Could you check a few things on this model? Use its own coordinates, in mm. Coordinates: 2 decimals unless noted, no trailing zeros. Order: outer loops, then holes, each group sorted by start corner. A loop starts at its lowest first (then second) coordinate and runs counter-clockwise, first axis right, second up. Notation, with made-up numbers: (86, 8) - (112, 8) arc R38 ccw to (112, 47) - close; hole circle Ø7 at (79.5, -3.75). An arc over 180 degrees is marked (long way). One line per item, written item: value.
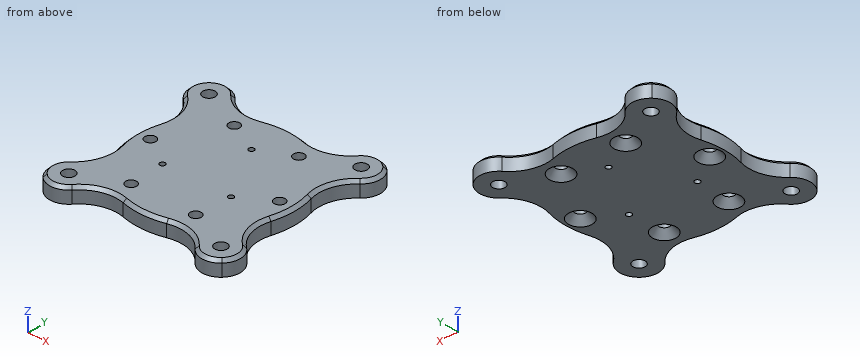
from build123d import *

# Parameters (mm, degrees)
SKETCH1_R                                      = 53.975
BOSS_EXTRUDE1_DEPTH                            = 6.35
CSK_FOR_8_FLAT_HEAD_MACHINE_SCREW1_D           = 4.4958
CSK_FOR_8_FLAT_HEAD_MACHINE_SCREW1_CSINK_D     = 9.7575878
CSK_FOR_8_FLAT_HEAD_MACHINE_SCREW1_CSINK_ANGLE = 82
CIRPATTERN1_COUNT                              = 6
F_10_CLEARANCE_HOLE1_D                         = 5.1054
CIRPATTERN2_COUNT                              = 4
F_4_40_TAPPED_HOLE1_D                          = 2.2606
CIRPATTERN3_COUNT                              = 3
CUT_EXTRUDE2_DEPTH                             = 77.59584682
CIRPATTERN4_COUNT                              = 4
CHAMFER1_SIZE                                  = 1.27


with BuildPart() as part:
    # Sketch1 → Boss-Extrude1 (new body)
    with BuildSketch(Plane.XY):
        Circle(SKETCH1_R)
    extrude(amount=BOSS_EXTRUDE1_DEPTH)

    # CSK for #8 Flat Head Machine Screw1 (through all)
    with Locations(Plane(origin=(0, 0, 0), x_dir=(-1, 0, 0), z_dir=(0, 0, -1))):
        with Locations((-13.49375, 23.371860585)):
            csk_for_8_flat_head_machine_screw1 = CounterSinkHole(CSK_FOR_8_FLAT_HEAD_MACHINE_SCREW1_D / 2, CSK_FOR_8_FLAT_HEAD_MACHINE_SCREW1_CSINK_D / 2, counter_sink_angle=CSK_FOR_8_FLAT_HEAD_MACHINE_SCREW1_CSINK_ANGLE)

    # CirPattern1: CSK for #8 Flat Head Machine Screw1 ×6 about axis
    cirpattern1_axis = Axis((0, 0, 0), (0, 0, 1))
    for i in range(1, CIRPATTERN1_COUNT):
        add(csk_for_8_flat_head_machine_screw1.rotate(cirpattern1_axis, i * 360 / CIRPATTERN1_COUNT), mode=Mode.SUBTRACT)

    # #10 Clearance Hole1 (through all)
    with Locations(Plane.XY.offset(6.35)):
        with Locations((31.75, 31.75)):
            f_10_clearance_hole1 = Hole(F_10_CLEARANCE_HOLE1_D / 2)

    # CirPattern2: #10 Clearance Hole1 ×4 about axis
    cirpattern2_axis = Axis((0, 0, 0), (0, 0, 1))
    for i in range(1, CIRPATTERN2_COUNT):
        add(f_10_clearance_hole1.rotate(cirpattern2_axis, i * 360 / CIRPATTERN2_COUNT), mode=Mode.SUBTRACT)

    # #4-40 Tapped Hole1 (through all)
    with Locations(Plane.XY.offset(6.35)):
        with Locations((0, 16.51)):
            f_4_40_tapped_hole1 = Hole(F_4_40_TAPPED_HOLE1_D / 2)

    # CirPattern3: #4-40 Tapped Hole1 ×3 about axis
    cirpattern3_axis = Axis((0, 0, 0), (0, 0, 1))
    for i in range(1, CIRPATTERN3_COUNT):
        add(f_4_40_tapped_hole1.rotate(cirpattern3_axis, i * 360 / CIRPATTERN3_COUNT), mode=Mode.SUBTRACT)

    # Sketch9 → Cut-Extrude2 (cut, through all)
    with BuildSketch(Plane(origin=(0, 0, 0), x_dir=(-1, 0, 0), z_dir=(0, 0, -1))):
        with BuildLine():
            Line((-37.362660076, 37.362660076), (-38.166088515, 38.166088515))
            ThreePointArc((-38.166088515, 38.166088515), (0, 53.975), (38.166088515, 38.166088515))
            Line((38.166088515, 38.166088515), (37.362660076, 37.362660076))
            ThreePointArc((37.362660076, 37.362660076), (31.392484898, 39.679444445), (25.65502333, 36.834797503))
            ThreePointArc((25.65502333, 36.834797503), (18.130045784, 31.830282128), (9.09329402, 31.74322611))
            ThreePointArc((9.09329402, 31.74322611), (0, 33.02), (-9.09329402, 31.74322611))
            ThreePointArc((-9.09329402, 31.74322611), (-18.130045784, 31.830282128), (-25.65502333, 36.834797503))
            ThreePointArc((-25.65502333, 36.834797503), (-31.392484898, 39.679444445), (-37.362660076, 37.362660076))
        make_face()
    cut_extrude2 = extrude(amount=-CUT_EXTRUDE2_DEPTH, mode=Mode.SUBTRACT)

    # CirPattern4: Cut-Extrude2 ×4 about axis
    cirpattern4_axis = Axis((0, 0, 0), (0, 0, 1))
    for i in range(1, CIRPATTERN4_COUNT):
        add(cut_extrude2.rotate(cirpattern4_axis, i * 360 / CIRPATTERN4_COUNT), mode=Mode.SUBTRACT)

    # Chamfer1
    chamfer1_edges = [part.edges().sort_by_distance(p)[0] for p in [
        (37.362660076, 37.362660076, 6.35),
        (-37.362660076, 37.362660076, 6.35),
        (-18.130045784, 31.830282128, 6.35),
        (0, 33.02, 6.35),
        (18.130045784, 31.830282128, 6.35),
        (37.362660076, -37.362660076, 6.35),
        (31.830282128, 18.130045784, 6.35),
        (33.02, 0, 6.35),
        (31.830282128, -18.130045784, 6.35),
        (-37.362660076, -37.362660076, 6.35),
        (18.130045784, -31.830282128, 6.35),
        (0, -33.02, 6.35),
        (-18.130045784, -31.830282128, 6.35),
        (-31.830282128, -18.130045784, 6.35),
        (-33.02, 0, 6.35),
        (-31.830282128, 18.130045784, 6.35),
    ]]
    chamfer(chamfer1_edges, length=CHAMFER1_SIZE)


solid = part.part
Item 1: I'm going to push flat-ended pins straight in: pin 1 Ø4.5 at (x, y) = (-31.75, 31.75) entering from +Z; pin 2 Ø1.5 at (x, z) = (-9, 5) entering from +Y; pin 3 Ø1.5 at (x, z) = (7.5, 0.5) entering from +Y; pin 4 Ø6 at (x, y) = (-26.99, 0) entering from -Z. Where does each tip first touch, or does it pass through?
Conclusion:
pin 1: through
pin 2: y = 31.97
pin 3: y = 32.32
pin 4: z = 2.16
Item 2: I want a section at B-B on z = 1.75. Give the number of separate pieces and of enclosed holes in the cut face, then the cut area to 3 significant figures.
Conclusion:
separate pieces: 1
enclosed holes: 13
area: 4,420 mm²
Item 3: I want a section at A-A on x = 0. Please give me the cut outline in (y, z).
Conclusion:
outline: (-33.02, 0) - (15.38, 0) - (15.38, 6.35) - (-31.75, 6.35) - (-33.02, 5.08) - close; (17.64, 0) - (33.02, 0) - (33.02, 5.08) - (31.75, 6.35) - (17.64, 6.35) - close
Item 4: If I drill on probe 1 along Y at (x, z) = (-30, 1); probe 2 along Y at (x, z) = (-30, 1.75); probe 3 along X at (y, z) = (30.5, 3.75), over which ranges is the centre line in solid material (lowest first)?
Conclusion:
probe 1: -39.49 to -33.61, -29.89 to -2.65, 2.65 to 29.89, 33.61 to 39.49
probe 2: -39.49 to -33.61, -29.89 to -1.48, 1.48 to 29.89, 33.61 to 39.49
probe 3: -39.59 to -33.98, -29.52 to 29.52, 33.98 to 39.59
